Check sheet for the modelled part. Datum: model origin and axes. Units: mm. Round coordinates to 2 decimals unless told otherwise and drop trailing zeros. Write each loop counter-clockwise with the first axis right and the second up, starting at its lowest first coordinate (ties: lowest second). Pieces come first, ordered by that corner, then holes. Notation, with made-up numbers: M 12.25,19.5 L 17.25,19.5 A22 cw 17.25,45.5 Z; hole C -9,74 d2. An arc over 180 degrees is marked long. One line per item, written item: value.
from build123d import *

# Parameters (mm, degrees)
CROQUIS1_W              = 400
CROQUIS1_H              = 450
CROQUIS1_R              = 3
CROQUIS1_W_2            = 320
CROQUIS1_H_2            = 350
SALIENTE_EXTRUIR1_DEPTH = 5
CHAFL_N1_SIZE           = 2


with BuildPart() as part:
    # Croquis1 → Saliente-Extruir1 (new body)
    with BuildSketch(Plane(origin=(0, 0, 0), x_dir=(1, 0, 0), z_dir=(0, 1, 0))):
        with Locations((27.104186234, -42.071984436)):
            Rectangle(CROQUIS1_W, CROQUIS1_H)
        with Locations(Location((-157.895813766, 132.928015564, 0), (0, 0, 270))):
            Circle(CROQUIS1_R, mode=Mode.SUBTRACT)
        with Locations(Location((-157.895813766, -237.071984436, 0), (0, 0, 270))):
            Circle(CROQUIS1_R, mode=Mode.SUBTRACT)
        with Locations(Location((212.104186234, -237.071984436, 0), (0, 0, 270))):
            Circle(CROQUIS1_R, mode=Mode.SUBTRACT)
        with Locations(Location((212.104186234, 132.928015564, 0), (0, 0, 270))):
            Circle(CROQUIS1_R, mode=Mode.SUBTRACT)
        with Locations(Location((-157.895813766, -27.071984436, 0), (0, 0, 270))):
            Circle(CROQUIS1_R, mode=Mode.SUBTRACT)
        with Locations(Location((212.104186234, -27.071984436, 0), (0, 0, 270))):
            Circle(CROQUIS1_R, mode=Mode.SUBTRACT)
        with Locations(Location((-72.895813766, 167.928015564, 0), (0, 0, 270))):
            Circle(CROQUIS1_R, mode=Mode.SUBTRACT)
        with Locations(Location((127.104186234, 167.928015564, 0), (0, 0, 270))):
            Circle(CROQUIS1_R, mode=Mode.SUBTRACT)
        with Locations(Location((127.104186234, -252.071984436, 0), (0, 0, 90))):
            Circle(CROQUIS1_R, mode=Mode.SUBTRACT)
        with Locations(Location((-72.895813766, -252.071984436, 0), (0, 0, 90))):
            Circle(CROQUIS1_R, mode=Mode.SUBTRACT)
        with Locations((27.104186234, -42.071984436)):
            Rectangle(CROQUIS1_W_2, CROQUIS1_H_2, mode=Mode.SUBTRACT)
    extrude(amount=SALIENTE_EXTRUIR1_DEPTH)

    # Chaflán1
    chafl_n1_edges = [part.edges().sort_by_distance(p)[0] for p in [
        (227.104186234, 5, 42.071984436),
        (27.104186234, 5, -182.928015564),
        (-172.895813766, 5, 42.071984436),
        (27.104186234, 5, 267.071984436),
    ]]
    chamfer(chafl_n1_edges, length=CHAFL_N1_SIZE)


solid = part.part
Q1. Sectioned sample at A-A on z = 145. Enter the section's corners in (x, y), and give its area (3 significant figures).
Completed:
outline: M -172.9,0 L -132.9,0 L -132.9,5 L -170.9,5 L -172.9,3 Z; M 187.1,0 L 227.1,0 L 227.1,3 L 225.1,5 L 187.1,5 Z
area: 396 mm^2
Q2. Depth check by flat-ended pin: P1, Ø3.5, axis at x = -72.9, z = -167.93, coming from the -Y side. Enter the tip coordinate at first touch or a pass-through.
Completed:
P1: through
Q3. Scan lines: line 1 (Z direction, x = 148, y = 1.95); line 2 (X direction, y = 2.2, z = -101.5); line 3 (X direction, y = 3.1, z = 140). Record each from-to range of solid material in increasing order. Write a range as [from, to].
Completed:
line 1: [-182.93, -132.93], [217.07, 267.07]
line 2: [-172.9, -132.9], [187.1, 227.1]
line 3: [-172.8, -132.9], [187.1, 227]
Q4. Sectioned sample at B-B on x = -49.5. Enter the section's corners in (y, z).
Completed:
outline: M 0,-182.93 L 3,-182.93 L 5,-180.93 L 5,-132.93 L 0,-132.93 Z; M 0,217.07 L 5,217.07 L 5,265.07 L 3,267.07 L 0,267.07 Z
Q5. Sectioned sample at C-C on y = 1.05. State how many separate pieces and enclosed holes the cut face has, and give its area (3 significant figures).
Completed:
separate pieces: 1
enclosed holes: 11
area: 67,700 mm^2
